Could you check a few things on this model? Use its own coordinates, in mm. A direction names the side the tool comes from. Round coordinates to 2 decimals unless told otherwise and drop trailing zeros. Write each loop counter-clockwise with the first axis right and the second up, starting at its lowest first coordinate (ties: lowest second). Pieces come first, ordered by that corner, then holes. Notation, with made-up numbers: M 21.25,72.5 L 48.25,72.5 A28 cw 48.25,90.5 Z; hole C 66,55.5 d3. An arc over 180 degrees is marked long. One line per item, written item: value. Start each with the question number.
(1) I want a section at A-A on z = -11. Count the separate pieces of the cut face and the enclosed holes in it, and give its area (3 significant figures).
(2) I'm going to push flat-ended pins straight in: pin 1 Ø11 at (x, z) = (135.5, -2) entering from -Y; pin 2 Ø2.5 at (y, z) = (-224.5, -24.5) entering from -X; pin 3 Ø2 at (x, y) = (121.5, -193.5) entering from -Z; pin 4 Ø21.5 at (y, z) = (-102, -14) entering from +X. Where does each tip first touch, or does it pass through?
(3) I want a section at C-C on y = -50. Please give me the cut outline in (x, z), and give its area (3 significant figures).
(4) Which directions (+Z, -Z, +X, -X, +Y, -Y) give clear straight access to the entire face, cutting with the end or side of a thin tool? Please do faces 1 (the face through (120.107, -109, -6)), 2 (the face through (-6, -218.958, -15)), 3 (the face through (-7, -222.755, -15)), 4 (the face through (-60, 3.048, 2)).
(5) Thinking about a two-plate mould opening in X: for faces 5 (the face through (-30, 5, 30)), 6 (the face through (130.99, 4.92, 22.46)), 7 (the face through (-66.38, 4.92, 32.43)), 8 (the face through (-60, 6.846, 2)), which applies, released by +X, released by -X, zero draft, split by the parting line, or undercut?
(6) If I drill on L1, parallel to Y at x = 77.5, z = -4.5 (3 decimals); L2, parallel to X at y = -150, z = 1.5; L3, parallel to Z at x = -2, y = 4, over which ranges is the centre line in solid material (lowest first)?
(7) I want a section at B-B on y = -135.5. Please give me the cut outline in (x, z).
```python
from build123d import *

# Parameters (mm, degrees)
SKETCH1_W                    = 75
SKETCH1_H                    = 75
BASE_FLANGE1_DEPTH           = 3.7973
EDGE_FLANGE1_STRIP_W         = 22.8092
EDGE_FLANGE1_STRIP_H         = 3.7973
EDGE_FLANGE1_STRIP_CUT_DEPTH = 75
EDGE_FLANGE1_DEPTH           = 75
EDGE_FLANGE2_STRIP_W         = 22.8092
EDGE_FLANGE2_STRIP_H         = 3.7973
EDGE_FLANGE2_STRIP_CUT_DEPTH = 75
EDGE_FLANGE2_DEPTH           = 75
EDGE_FLANGE3_DEPTH           = 214.38618
EDGE_FLANGE3_START           = -3.7973
EDGE_FLANGE3_FLAT_DEPTH      = 3.7973
EDGE_FLANGE4_DEPTH           = 71.19
EDGE_FLANGE5_DEPTH           = 36.19
BREAK_CORNER1_START          = -222.755
BREAK_CORNER1_DEPTH          = 3.7973
BREAK_CORNER2_START          = -74.246212025
BREAK_CORNER2_OUTLINE_W      = 51.869221049
BREAK_CORNER2_OUTLINE_H      = 3.7973
BREAK_CORNER2_DEPTH          = 7.071067812
BREAK_CORNER2_START_2        = -30.978348084
BREAK_CORNER2_2_OUTLINE_W    = 7.130778951
BREAK_CORNER2_2_OUTLINE_H    = 3.7973
BREAK_CORNER2_2_DEPTH        = 14.142135624
M8_CLEARANCE_HOLE1_D         = 9
M8_CLEARANCE_HOLE1_DEPTH     = 13
M8_CLEARANCE_HOLE1_TIP       = 2.703872786
BREAK_CORNER3_START          = 3.04848
BREAK_CORNER3_DEPTH          = 3.7973
M8_START                     = -226.945
M8_CLEARANCE_SLOT1_DEPTH     = 7.9873


# Read off the part's stored shape, not the designer's step: Break-Corner1, Break-Corner2, Break-Corner3, M8 Clearance Slot1
# Sheet-metal steps are written as plain solids
with BuildPart() as part:
    # Sketch1 → Base-Flange1 (new body)
    with BuildSketch(Plane(origin=(0, 6.84578, 0), x_dir=(1, 0, 0), z_dir=(0, 1, 0))):
        Rectangle(SKETCH1_W, SKETCH1_H)
    extrude(amount=-BASE_FLANGE1_DEPTH)

    # Edge-Flange1 strip (across the edge) → Edge-Flange1 strip cut (cut)
    with BuildSketch(Plane(origin=(-37.5, 3.04848, -37.5), x_dir=(0, 0, 1), z_dir=(1, 0, 0))):
        with Locations((-7.5946, -1.89865)):
            Rectangle(EDGE_FLANGE1_STRIP_W, EDGE_FLANGE1_STRIP_H)
    extrude(amount=EDGE_FLANGE1_STRIP_CUT_DEPTH, mode=Mode.SUBTRACT)

    # Edge-Flange1 section (across the edge) → Edge-Flange1 (add)
    with BuildSketch(Plane(origin=(-37.5, 3.04848, -37.5), x_dir=(0, 0, 1), z_dir=(1, 0, 0))):
        with BuildLine():
            Line((-3.7973, 3.81), (-3.7973, 229.99348))
            Line((-3.7973, 229.99348), (0, 229.99348))
            Line((0, 229.99348), (0, 3.81))
            ThreePointArc((0, 3.81), (1.115923164, 1.115923164), (3.81, 0))
            Line((3.81, 0), (3.81, -3.7973))
            ThreePointArc((3.81, -3.7973), (-1.569173417, -1.569173417), (-3.7973, 3.81))
        make_face()
    extrude(amount=EDGE_FLANGE1_DEPTH)

    # Edge-Flange2 strip (across the edge) → Edge-Flange2 strip cut (cut)
    with BuildSketch(Plane(origin=(-37.5, -226.945, -37.5), x_dir=(0, 1, 0), z_dir=(1, 0, 0))):
        with Locations((-3.7973, -1.89865)):
            Rectangle(EDGE_FLANGE2_STRIP_W, EDGE_FLANGE2_STRIP_H)
    extrude(amount=EDGE_FLANGE2_STRIP_CUT_DEPTH, mode=Mode.SUBTRACT)

    # Edge-Flange2 section (across the edge) → Edge-Flange2 (add)
    with BuildSketch(Plane(origin=(-37.5, -226.945, -37.5), x_dir=(0, 1, 0), z_dir=(1, 0, 0))):
        with BuildLine():
            Line((0, 3.81), (0, 40))
            Line((0, 40), (3.7973, 40))
            Line((3.7973, 40), (3.7973, 3.81))
            ThreePointArc((3.7973, 3.81), (4.913223164, 1.115923164), (7.6073, 0))
            Line((7.6073, 0), (7.6073, -3.7973))
            ThreePointArc((7.6073, -3.7973), (2.228126583, -1.569173417), (0, 3.81))
        make_face()
    extrude(amount=EDGE_FLANGE2_DEPTH)

    # Edge-Flange3 bend section (across the edge) → Edge-Flange3 (add)
    with BuildSketch(Plane(origin=(-41.31, -0.76152, -37.5), x_dir=(1, 0, 0), z_dir=(0, -1, 0))):
        with BuildLine():
            Line((-3.7973, 3.81), (0, 3.81))
            ThreePointArc((0, 3.81), (1.115923164, 1.115923164), (3.81, 0))
            Line((3.81, 0), (3.81, -3.7973))
            ThreePointArc((3.81, -3.7973), (-1.569173417, -1.569173417), (-3.7973, 3.81))
        make_face()
    extrude(amount=EDGE_FLANGE3_DEPTH)

    # Edge-Flange3 profile (on flange) → Edge-Flange3 flat (add)
    with BuildSketch(Plane(origin=(-41.31, 0, -37.5), x_dir=(0, 1, 0), z_dir=(1, 0, 0)).offset(EDGE_FLANGE3_START)):
        Polygon((-215.1477, 3.81), (-0.76152, 3.81), (-0.76152, 75), (-215.1477, 40), align=None)
    extrude(amount=EDGE_FLANGE3_FLAT_DEPTH)

    # Edge-Flange4 section (across the edge) → Edge-Flange4 (add)
    with BuildSketch(Plane(origin=(-45.1073, 3.04848, 37.5), x_dir=(0, -1, 0), z_dir=(0, 0, -1))):
        with BuildLine():
            Line((-3.7973, 3.81), (-3.7973, 26.2027))
            Line((-3.7973, 26.2027), (0, 26.2027))
            Line((0, 26.2027), (0, 3.81))
            ThreePointArc((0, 3.81), (1.115923164, 1.115923164), (3.81, 0))
            Line((3.81, 0), (3.81, -3.7973))
            ThreePointArc((3.81, -3.7973), (-1.569173417, -1.569173417), (-3.7973, 3.81))
        make_face()
    extrude(amount=EDGE_FLANGE4_DEPTH)

    # Edge-Flange5 section (across the edge) → Edge-Flange5 (add)
    with BuildSketch(Plane(origin=(-41.31, -218.9577, 2.5), x_dir=(0, 1, 0), z_dir=(0, 0, -1))):
        with BuildLine():
            Line((-3.7973, 3.81), (-3.7973, 66.2027))
            Line((-3.7973, 66.2027), (0, 66.2027))
            Line((0, 66.2027), (0, 3.81))
            ThreePointArc((0, 3.81), (1.115923164, 1.115923164), (3.81, 0))
            Line((3.81, 0), (3.81, -3.7973))
            ThreePointArc((3.81, -3.7973), (-1.569173417, -1.569173417), (-3.7973, 3.81))
        make_face()
    extrude(amount=EDGE_FLANGE5_DEPTH)

    # Break-Corner1 outline → Break-Corner1 (cut)
    with BuildSketch(Plane(origin=(0, 0, 0), x_dir=(1, 0, 0), z_dir=(0, 1, 0)).offset(BREAK_CORNER1_START)):
        Polygon((24.8927, -2.5), (24.8927, 7.5), (14.8927, -2.5), align=None)
        Polygon((14.8927, 33.69), (24.8927, 23.69), (24.8927, 33.69), align=None)
    extrude(amount=BREAK_CORNER1_DEPTH, mode=Mode.SUBTRACT)

    # Break-Corner2 outline → Break-Corner2 (cut)
    with BuildSketch(Plane(origin=(0, 0, 0), x_dir=(0.707106781186549, 0, -0.707106781186546), z_dir=(0.707106781186546, 0, 0.707106781186549)).offset(BREAK_CORNER2_START)):
        with Locations((-43.934610525, 4.94713)):
            Rectangle(BREAK_CORNER2_OUTLINE_W, BREAK_CORNER2_OUTLINE_H)
    extrude(amount=BREAK_CORNER2_DEPTH, mode=Mode.SUBTRACT)

    # Break-Corner2 2 outline → Break-Corner2 2 (cut)
    with BuildSketch(Plane(origin=(0, 0, 0), x_dir=(0.707106781186549, 0, -0.707106781186546), z_dir=(0.707106781186546, 0, 0.707106781186549)).offset(BREAK_CORNER2_START_2)):
        with Locations((-73.434610525, 4.94713)):
            Rectangle(BREAK_CORNER2_2_OUTLINE_W, BREAK_CORNER2_2_OUTLINE_H)
    extrude(amount=BREAK_CORNER2_2_DEPTH, mode=Mode.SUBTRACT)

    # M8 Clearance Hole1
    with Locations(Plane(origin=(0, 6.84578, 0), x_dir=(1, 0, 0), z_dir=(0, 1, 0))):
        with Locations((-2.5, -19.962925734), (-2.5, 20.037074266), (-59.31, -25.5)):
            Hole(M8_CLEARANCE_HOLE1_D / 2, depth=M8_CLEARANCE_HOLE1_DEPTH)
            with Locations((0, 0, -(M8_CLEARANCE_HOLE1_DEPTH + M8_CLEARANCE_HOLE1_TIP / 2))):  # 118° drill point
                Cone(0, M8_CLEARANCE_HOLE1_D / 2, M8_CLEARANCE_HOLE1_TIP, mode=Mode.SUBTRACT)

    # Mirror1: part across plane


with BuildPart() as part_1:
    add(part.part)
    add(part.part.mirror(Plane(origin=(37.5, 3.04848, -41.2973), x_dir=(0, 0, 1), z_dir=(1, 0, 0))))

    # Break-Corner3 outline → Break-Corner3 (cut)
    with BuildSketch(Plane(origin=(0, 0, 0), x_dir=(1, 0, 0), z_dir=(0, 1, 0)).offset(BREAK_CORNER3_START)):
        Polygon((-37.5, -37.5), (-22.5, -37.5), (-37.5, -22.5), align=None)
        Polygon((112.5, -22.5), (97.5, -37.5), (112.5, -37.5), align=None)
    extrude(amount=BREAK_CORNER3_DEPTH, mode=Mode.SUBTRACT)

    # M8 Clearance Slot1 outline → M8 Clearance Slot1 (cut)
    with BuildSketch(Plane(origin=(0, 0, 0), x_dir=(1, 0, 0), z_dir=(0, 1, 0)).offset(M8_START)):
        with BuildLine():
            ThreePointArc((-0.9328125, 23.696875), (3.5671875, 19.196875), (8.0671875, 23.696875))
            Line((8.0671875, 23.696875), (8.0671875, 26.696875))
            ThreePointArc((8.0671875, 26.696875), (3.5671875, 31.196875), (-0.9328125, 26.696875))
            Line((-0.9328125, 26.696875), (-0.9328125, 23.696875))
        make_face()
        with BuildLine():
            ThreePointArc((66.9328125, 23.696875), (71.4328125, 19.196875), (75.9328125, 23.696875))
            Line((75.9328125, 23.696875), (75.9328125, 26.696875))
            ThreePointArc((75.9328125, 26.696875), (71.4328125, 31.196875), (66.9328125, 26.696875))
            Line((66.9328125, 26.696875), (66.9328125, 23.696875))
        make_face()
    extrude(amount=M8_CLEARANCE_SLOT1_DEPTH, mode=Mode.SUBTRACT)


solid = part_1.part
```
Found:
1. separate pieces: 4
1. enclosed holes: 0
1. area: 3,550 mm²
2. pin 1: stops at y = 3.05
2. pin 2: stops at x = -37.5
2. pin 3: passes through
2. pin 4: stops at x = 120.11
3. outline: M -45.11,-33.69 A7.61 ccw -37.5,-41.3 L 112.5,-41.3 A7.61 ccw 120.11,-33.69 L 120.11,29.46 L 116.31,29.46 L 116.31,-33.69 A3.81 cw 112.5,-37.5 L -37.5,-37.5 A3.81 cw -41.31,-33.69 L -41.31,29.46 L -45.11,29.46 Z
3. area: 1,120 mm²
4. face 1: +Z, -Z, +X, -Y
4. face 2: +Z
4. face 3: +Z, +X, -X
4. face 4: +Z, -Z, -X, -Y
5. face 5: undercut
5. face 6: undercut
5. face 7: released by -X
5. face 8: zero draft
6. L1: y = -226.945 to -223.148, -222.755 to -218.958, 3.048 to 6.846
6. L2: x = -45.11 to -41.31, 116.31 to 120.11
6. L3: z = -39.62 to -24.51, -15.56 to 15.49, 24.44 to 37.5
7. outline: M -45.11,-33.69 A7.61 ccw -37.5,-41.3 L 112.5,-41.3 A7.61 ccw 120.11,-33.69 L 120.11,15.5 L 116.31,15.5 L 116.31,-33.69 A3.81 cw 112.5,-37.5 L -37.5,-37.5 A3.81 cw -41.31,-33.69 L -41.31,15.5 L -45.11,15.5 Z
